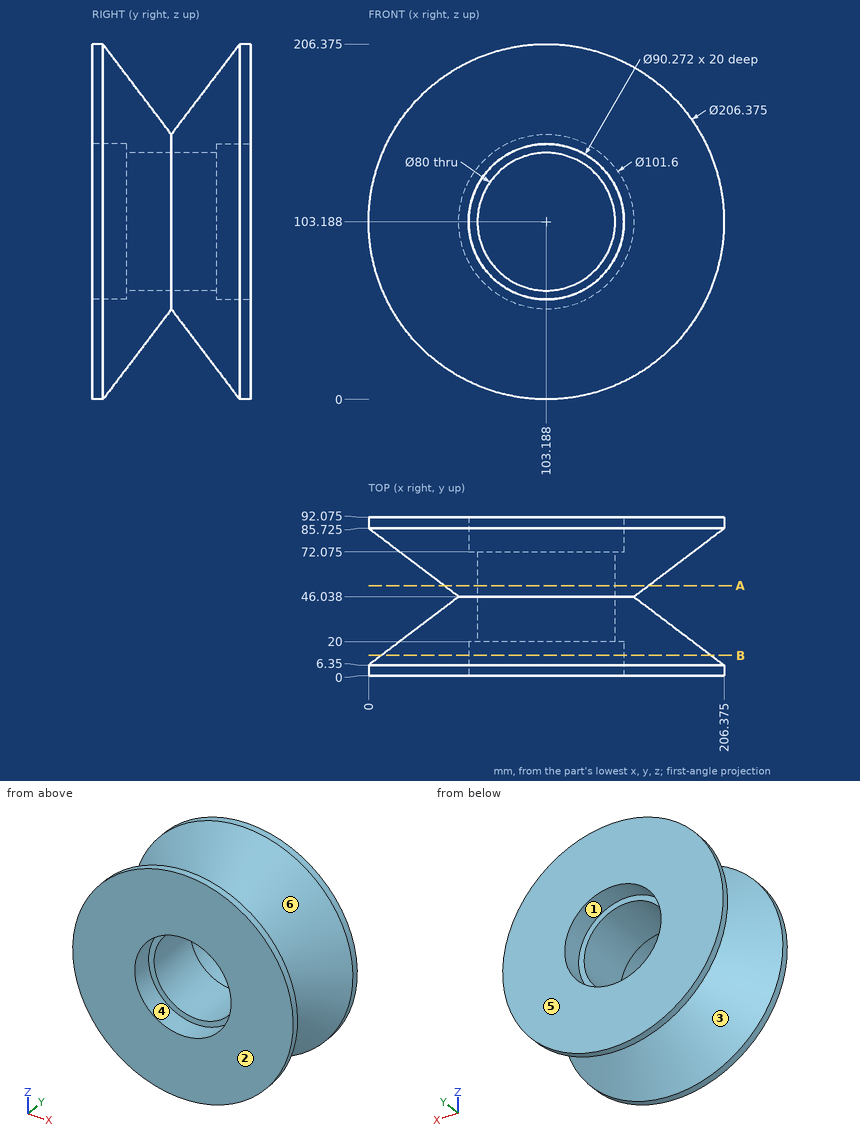
Design review of the part shown in the three views and the two pictorial views. Dimensions are in mm from the part's minimum x, y and z. A direction names the side the tool comes from. Round coordinates to 2 decimals unless told otherwise and drop trailing zeros. Loops run counter-clockwise (first coordinate to the right, second up) from the corner with the lowest first, then second, coordinate; pieces in that order, holes last. Notation, with made-up numbers: (88, 22.5) -> (137, 22.5) arc R12 ccw to (137, 37.5) -> close; hole circle Ø1 at (18.5, 83.5). An arc over 180 degrees is marked (long way). Return JSON: item names as keys, results as strings.
(1) The part is to be moulded in two halves that separate along Y. For the marked faces 4, 5 and 6, say which applies: released by +Y, released by -Y, zero draft, split by the parting line, or undercut.
Solved:
{"face 4": "zero draft", "face 5": "released by +Y", "face 6": "undercut"}
(2) For line 1 (Y direction, x = 61, z = 22) (1 decimal); line 2 (Z direction, x = 137, y = 55) (1 decimal); line 3 (Y direction, x = 140, z = 87) (1 decimal), list the stretches that pass through material, from the lowest coordinate up.
Solved:
{"line 1": "0 to 15.2, 76.9 to 92.1", "line 2": "50.5 to 81.8, 124.6 to 155.9", "line 3": "20 to 72.1"}
(3) Add section B-B on y = 12. Write out the cut boundary in (x, z) (1 decimal).
Solved:
{"outline": "circle Ø191.5 at (103.2, 103.2); hole circle Ø90.3 at (103.2, 103.2)"}
(4) For the marked faces 1, 2 and 3, list the 3-axis set-ups (+Z, -Z, +X, -X, +Y, -Y) from which the entire face can be reached by the end or side of a thin tool; tool diameter is ignored.
Solved:
{"face 1": "+Y", "face 2": "+Z, -Z, +X, -X, -Y", "face 3": "none"}
(5) Add section A-A on y = 52.5. Write out the cut boundary in (x, z), plus the area to 3 significant figures.
Solved:
{"outline": "circle Ø118.66 at (103.19, 103.19); hole circle Ø80 at (103.19, 103.19)", "area": "6,030 mm2"}
(6) For pin 1 (6 mm diameter, centred on y = 24, z = 114.5, fed in from -X) (1 decimal); pin 2 (6 mm diameter, centred on x = 119.5, y = 19, fed in from +Z); pin 3 (1.5 mm diameter, centred on x = 47.5, z = 181.5, fed in from -Y); pin 4 (8 mm diameter, centred on x = 131, y = 12.5, fed in from -Z) (1 decimal), all flat-tipped, find the tip position at first contact; note any pin that passes through.
Solved:
{"pin 1": "x = 20.1", "pin 2": "z = 192.19", "pin 3": "y = 0", "pin 4": "z = 6.7"}
